from build123d import *

# Parameters (mm, degrees)
F0_R     = 5.953125
F1_DEPTH = 4.7625


with BuildPart() as f1:
    # F0 (on Front) → F1 (new body)
    with BuildSketch(Plane.XZ):
        with BuildLine():
            Line((101.6, 4.7625), (101.6, 96.8375))
            Line((101.6, 96.8375), (71.4375, 96.8375))
            Line((71.4375, 96.8375), (66.675, 92.075))
            Line((66.675, 92.075), (66.675, 4.7625))
            ThreePointArc((66.675, 4.7625), (0, -61.9125), (-66.675, 4.7625))
            Line((-66.675, 4.7625), (-66.675, 92.075))
            Line((-66.675, 92.075), (-71.4375, 96.8375))
            Line((-71.4375, 96.8375), (-101.6, 96.8375))
            Line((-101.6, 96.8375), (-101.6, 4.7625))
            ThreePointArc((-101.6, 4.7625), (0, -96.8375), (101.6, 4.7625))
        make_face()
        with Locations((-39.6875, -74.786922)):
            Circle(F0_R, mode=Mode.SUBTRACT)
        with Locations((-87.471098, -11.1125)):
            Circle(F0_R, mode=Mode.SUBTRACT)
        with Locations((39.6875, -74.786922)):
            Circle(F0_R, mode=Mode.SUBTRACT)
        with Locations((87.471098, -11.1125)):
            Circle(F0_R, mode=Mode.SUBTRACT)
        with Locations((-88.9, 68.2625)):
            Circle(F0_R, mode=Mode.SUBTRACT)
        with Locations((88.9, 68.2625)):
            Circle(F0_R, mode=Mode.SUBTRACT)
    extrude(amount=F1_DEPTH)


solid = f1.part
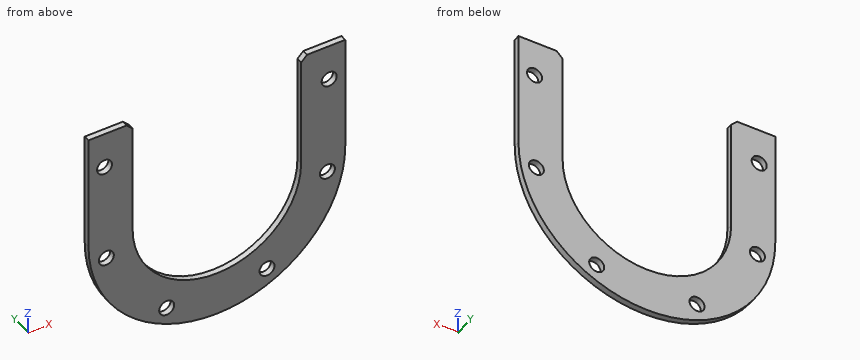
Could you check a few things on this model? Use its own coordinates, in mm. Coordinates: 2 decimals unless noted, no trailing zeros. Write each loop counter-clockwise with the first axis right and the second up, starting at its lowest first coordinate (ties: lowest second). Pieces come first, ordered by that corner, then holes. Notation, with made-up numbers: (1, 30.25) - (51, 30.25) arc R23 cw to (51, 60.25) - close; hole circle Ø2 at (29, -31.75). An arc over 180 degrees is marked (long way). Put each result on its own line as item: value. Start each with the question number.
Q1. I want a section at B-B on x = -88.9. Write out the boundary of the cut face in (y, z).
Q2. Please list where these lines run through material, in increasing order: L1, parallel to X at y = -0.5, z = 23.5 (3 decimals); L2, parallel to X at y = -1.1, z = 68.5 (3 decimals); L3, parallel to Z at x = -88.9, y = -3.3.
Q3. I want a section at A-A on z = 84.5. Write out the boundary of the cut face in (x, y) (1 decimal), plus the area to 3 significant figures.
Q4. I want a section at C-C on y = -3.85. Count the separate pieces of the cut face and the enclosed holes in it, plus the area to 3 significant figures.
Q5. I want a section at D-D on x = 0. Write out the boundary of the cut face in (y, z).
Q6. I'm going to push a flat-ended pin straight in: P1, Ø1.5, axis at x = -76, y = -1.5, coming from the -Z side. Where does the tip first touch, or does it pass through?
Checks:
1. outline: (-4.76, -44.42) - (0, -44.42) - (0, -16.89) - (-4.76, -16.89) - close; (-4.76, -5.33) - (0, -5.33) - (0, 62.31) - (-4.76, 62.31) - close; (-4.76, 74.22) - (0, 74.22) - (0, 96.84) - (-4.76, 96.84) - close
2. L1: -101.6 to -66.675, 66.675 to 101.6
2. L2: -101.6 to -94.848, -82.952 to -66.675, 66.675 to 82.952, 94.848 to 101.6
2. L3: -44.42 to -16.89, -5.33 to 62.31, 74.22 to 96.84
3. outline: (-101.6, -4.8) - (-66.7, -4.8) - (-66.7, 0) - (-101.6, 0) - close; (66.7, -4.8) - (101.6, -4.8) - (101.6, 0) - (66.7, 0) - close
3. area: 333 mm²
4. separate pieces: 1
4. enclosed holes: 6
4. area: 15,000 mm²
5. outline: (-4.76, -96.84) - (0, -96.84) - (0, -61.91) - (-4.76, -61.91) - close
6. P1: z = -63.5
